Here's how the part is built. I have some questions about the finished solid (model axes, mm). Give positions to 0.01 mm unless a question says otherwise; leave off trailing zeros. Loops run counter-clockwise (first coordinate to the right, second up) from the corner with the lowest first, then second, coordinate; pieces in that order, holes last. Notation, with made-up numbers: (-12.5, -1.5) - (23.5, -1.5) arc R27 cw to (23.5, 23.5) - close; hole circle Ø5 at (15.25, 2). An arc over 180 degrees is marked (long way). Put each result on its own line as item: value. Start each with the question number.
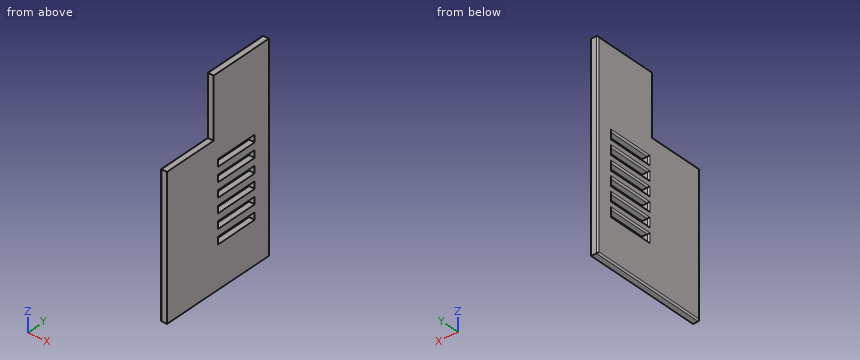
from build123d import *

# Parameters (mm, degrees)
BOSS_EXTRUDE1_DEPTH = 4.6
SKETCH2_W           = 42
SKETCH2_H           = 55
CUT_EXTRUDE1_DEPTH  = 139.94227549
SKETCH4_W           = 5
SKETCH4_H           = 30
CUT_EXTRUDE3_DEPTH  = 10
FILLET1_R           = 1


with BuildPart() as part:
    # Sketch1 → Boss-Extrude1 (new body)
    with BuildSketch(Plane(origin=(0, 0, 0), x_dir=(0, 0, -1), z_dir=(1, 0, 0))):
        Polygon((-27, 80.714285714), (113, 80.714285714), (113, -2.285714286), (13, -2.285714286), (13, -19.285714286), (-27, -19.285714286), align=None)
    extrude(amount=BOSS_EXTRUDE1_DEPTH)

    # Sketch2 → Cut-Extrude1 (cut, through all)
    with BuildSketch(Plane(origin=(4.6, 0, 0), x_dir=(0, 0, -1), z_dir=(1, 0, 0))):
        with Locations((-6, 8.214285714)):
            Rectangle(SKETCH2_W, SKETCH2_H)
    extrude(amount=-CUT_EXTRUDE1_DEPTH, mode=Mode.SUBTRACT)

    # Sketch4 → Cut-Extrude3 (cut)
    with BuildSketch(Plane.ZY):
        with Locations((-41.233318098, 54.194727162)):
            Rectangle(SKETCH4_W, SKETCH4_H)
        with Locations((-31.233318098, 54.194727162)):
            Rectangle(SKETCH4_W, SKETCH4_H)
        with Locations((-51.233318098, 54.194727162)):
            Rectangle(SKETCH4_W, SKETCH4_H)
        with Locations((-61.233318098, 54.194727162)):
            Rectangle(SKETCH4_W, SKETCH4_H)
        with Locations((-71.233318098, 54.194727162)):
            Rectangle(SKETCH4_W, SKETCH4_H)
        with Locations((-81.233318098, 54.194727162)):
            Rectangle(SKETCH4_W, SKETCH4_H)
    extrude(amount=-CUT_EXTRUDE3_DEPTH, mode=Mode.SUBTRACT)

    # Fillet1
    fillet1_edges = [part.edges().sort_by_distance(p)[0] for p in [
        (0, 39.194727162, -71.233318098),
        (0, 54.194727162, -68.733318098),
        (0, 69.194727162, -71.233318098),
        (0, 54.194727162, -73.733318098),
        (0, 39.194727162, -81.233318098),
        (0, 54.194727162, -78.733318098),
        (0, 69.194727162, -81.233318098),
        (0, 54.194727162, -83.733318098),
        (0, -2.285714286, -64),
        (0, 16.714285714, -15),
        (0, 35.714285714, 6),
        (0, 80.714285714, -43),
        (0, 39.214285714, -113),
        (0, 54.194727162, -28.733318098),
        (0, 69.194727162, -31.233318098),
        (0, 54.194727162, -33.733318098),
        (0, 39.194727162, -31.233318098),
        (0, 39.194727162, -41.233318098),
        (0, 54.194727162, -38.733318098),
        (0, 69.194727162, -41.233318098),
        (0, 54.194727162, -43.733318098),
        (0, 58.214285714, 27),
        (0, 39.194727162, -51.233318098),
        (0, 54.194727162, -48.733318098),
        (0, 69.194727162, -51.233318098),
        (0, 54.194727162, -53.733318098),
        (0, 39.194727162, -61.233318098),
        (0, 54.194727162, -58.733318098),
        (0, 69.194727162, -61.233318098),
        (0, 54.194727162, -63.733318098),
    ]]
    fillet(fillet1_edges, radius=FILLET1_R)


solid = part.part
1) Suppose I cut it at D-D on z = -2.5. Please give me the cut outline in (x, y), plus the area to 3 significant figures.
2) Suppose I cut it at A-A on x = 2.2. Give the number of separate pieces and of enclosed holes in the cut face, plus the area to 3 significant figures.
3) Suppose I cut it at B-B on y = 30.5. Please give me the cut outline in (x, z).
4) I'm going to push a flat-ended pin straight in: P1, Ø1.8, axis at x = 2.5, z = 14.5, coming from the -Y side. Where does the tip first touch, or does it pass through?
5) I need wall thicknesses on line 1 (Z direction, x = 1.55, y = 33); line 2 (Y direction, x = 2.1, z = 0); line 3 (Y direction, x = 0.35, z = -49). Which ranges of each line are inside material? Lowest first, please.
Ans:
1. outline: (0, 36.71) arc R1 ccw to (1, 35.71) - (4.6, 35.71) - (4.6, 80.71) - (1, 80.71) arc R1 ccw to (0, 79.71) - close
1. area: 207 mm²
2. separate pieces: 1
2. enclosed holes: 6
2. area: 9,120 mm²
3. outline: (0, -112) arc R1 ccw to (1, -113) - (4.6, -113) - (4.6, -15) - (1, -15) arc R1 ccw to (0, -16) - close
4. P1: stops at y = 35.71
5. line 1: z = -113 to -15
5. line 2: y = 35.71 to 80.71
5. line 3: y = -2.05 to 38.95, 69.43 to 80.47
